Here's how the part is built. I have some questions about the finished solid (model axes, mm). Coordinates: 2 decimals unless noted, no trailing zeros. Order: outer loops, then holes, each group sorted by start corner. A loop starts at its lowest first (then second) coordinate and runs counter-clockwise, first axis right, second up. Notation, with made-up numbers: (5.5, -40) - (23.5, -40) arc R23 cw to (23.5, -31) - close; hole circle Ø1 at (-24, 38). An arc over 180 degrees is marked (long way). Answer as CSV lines item,"result". Start each with the question number.
Item 1: Imagine slicing it at A-A on x = 12.7. List the corners of the cut face in (y, z) for me, and give its area (3 significant figures).
Item 2: I need wall thicknesses on line 1 (Y direction, x = 12.7, z = 139); line 2 (X direction, y = 23.25, z = 264); line 3 (X direction, y = 16.75, z = 201) (3 decimals). Which ranges of each line are inside material? Lowest first, please.
Item 3: I'm going to push flat-ended pins straight in: pin 1 (5 mm diameter, centred on x = 12, z = 168.5, fed in from +Y); pin 2 (3 mm diameter, centred on y = 12.5, z = 186.5, fed in from +X); pin 3 (1.8 mm diameter, centred on y = 11.5, z = 166, fed in from -X). Where does each tip first touch, or does it pass through?
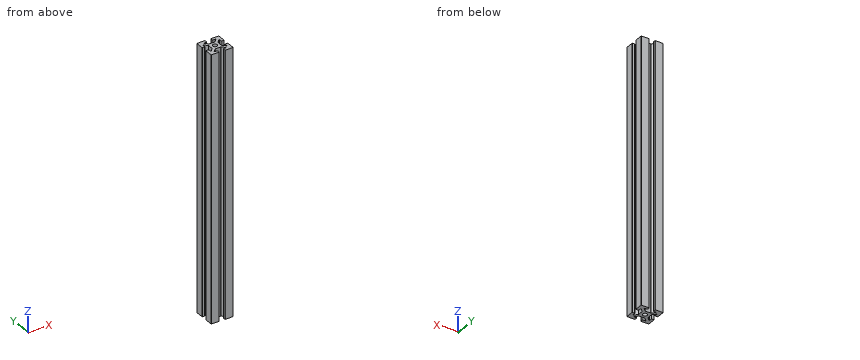
Autodesk Inventor part; units mm, degrees
ref_plane "YZ Plane" through (0, 0, 0) normal (1, 0, 0) x (0, 1, 0)
ref_plane "XZ Plane" through (0, 0, 0) normal (0, 1, 0) x (-1, 0, 0)
ref_plane "XY Plane" through (0, 0, 0) normal (0, 0, 1) x (1, 0, 0)
sketch "Sketch1" plane through (0, 0, 0) normal (0, 0, 1) x (1, 0, 0)
  line L0 (0, 0) -> (25.4, 0) construction
  line L1 (25.4, 0) -> (25.4, 25.4) construction
  line L2 (25.4, 25.4) -> (0, 25.4) construction
  line L3 (0, 25.4) -> (0, 0) construction
  line L4 (0, 25.4) -> (9.4615, 25.4) construction
  line L5 (9.4615, 25.4) -> (9.4615, 15.9385) construction
  line L6 (9.4615, 15.9385) -> (0, 15.9385) construction
  line L7 (0, 15.9385) -> (0, 25.4) construction
  line L8 (25.4, 25.4) -> (15.9385, 25.4) construction
  line L9 (15.9385, 25.4) -> (15.9385, 15.9385) construction
  line L10 (15.9385, 15.9385) -> (25.4, 15.9385) construction
  line L11 (25.4, 15.9385) -> (25.4, 25.4) construction
  line L12 (25.4, 0) -> (15.9385, 0) construction
  line L13 (15.9385, 0) -> (15.9385, 9.4615) construction
  line L14 (15.9385, 9.4615) -> (25.4, 9.4615) construction
  line L15 (25.4, 9.4615) -> (25.4, 0) construction
  line L16 (0, 0) -> (9.4615, 0) construction
  line L17 (9.4615, 0) -> (9.4615, 9.4615) construction
  line L18 (9.4615, 9.4615) -> (0, 9.4615) construction
  line L19 (0, 9.4615) -> (0, 0) construction
  circle A0 centre (12.7, 12.7) radius 2.5797
  line L20 (0, 25.4) -> (9.4615, 25.4)
  line L21 (9.4615, 25.4) -> (9.4615, 22.225)
  line L22 (0, 25.4) -> (0, 15.9385)
  line L23 (0, 15.9385) -> (3.175, 15.9385)
  line L24 (0, 0) -> (0, 9.4615)
  line L25 (0, 9.4615) -> (3.175, 9.4615)
  line L26 (0, 0) -> (9.4615, 0)
  line L27 (9.4615, 0) -> (9.4615, 3.175)
  line L28 (25.4, 0) -> (15.9385, 0)
  line L29 (25.4, 0) -> (25.4, 9.4615)
  line L30 (25.4, 9.4615) -> (22.225, 9.4615)
  line L31 (15.9385, 0) -> (15.9385, 3.175)
  line L32 (25.4, 25.4) -> (25.4, 15.9385)
  line L33 (25.4, 25.4) -> (15.9385, 25.4)
  line L34 (15.9385, 25.4) -> (15.9385, 22.225)
  line L35 (25.4, 15.9385) -> (22.225, 15.9385)
  line L36 (9.4615, 22.225) -> (5.2705, 22.225)
  line L37 (3.175, 15.9385) -> (3.175, 20.1295)
  line L38 (3.175, 9.4615) -> (3.175, 5.2705)
  line L39 (9.4615, 3.175) -> (5.2705, 3.175)
  line L40 (15.9385, 3.175) -> (20.1295, 3.175)
  line L41 (22.225, 9.4615) -> (22.225, 5.2705)
  line L42 (15.9385, 22.225) -> (20.1295, 22.225)
  line L43 (22.225, 15.9385) -> (22.225, 20.1295)
  line L44 (7.3422, 7.3422) -> (18.0578, 7.3422) construction
  line L45 (18.0578, 7.3422) -> (18.0578, 18.0578) construction
  line L46 (18.0578, 18.0578) -> (7.3422, 18.0578) construction
  line L47 (7.3422, 18.0578) -> (7.3422, 7.3422) construction
  line L48 (7.3422, 7.3422) -> (18.0578, 18.0578) construction
  line L49 (18.0578, 7.3422) -> (7.3422, 18.0578) construction
  line L50 (5.2705, 22.225) -> (9.4615, 18.0578)
  line L51 (3.175, 20.1295) -> (7.3422, 15.9385)
  line L52 (20.1295, 22.225) -> (15.9385, 18.0578)
  line L53 (22.225, 20.1295) -> (18.0578, 15.9385)
  line L54 (22.225, 5.2705) -> (18.0578, 9.4615)
  line L55 (20.1295, 3.175) -> (15.9385, 7.3422)
  line L56 (5.2705, 3.175) -> (9.4615, 7.3422)
  line L57 (3.175, 5.2705) -> (7.3422, 9.4615)
  line L58 (7.3422, 15.9385) -> (7.3422, 9.4615)
  line L59 (9.4615, 18.0578) -> (15.9385, 18.0578)
  line L60 (18.0578, 15.9385) -> (18.0578, 9.4615)
  line L61 (15.9385, 7.3422) -> (9.4615, 7.3422)
  dimension "d0" = 25.4
  dimension "d1" = 25.4
  dimension "d2" = 9.4615
  dimension "d3" = 9.4615
  dimension "d4" = 9.4615
  dimension "d5" = 9.4615
  dimension "d6" = 9.4615
  dimension "d7" = 9.4615
  dimension "d8" = 9.4615
  dimension "d9" = 9.4615
  dimension "d10" = 12.7
  dimension "d11" = 12.7
  dimension "d12" = 5.1594
  dimension "d13" = 3.175
  dimension "d14" = 3.175
  dimension "d15" = 3.175
  dimension "d16" = 3.175
  dimension "d17" = 3.175
  dimension "d18" = 3.175
  dimension "d19" = 3.175
  dimension "d20" = 3.175
  dimension "d21" = 4.191
  dimension "d22" = 4.191
  dimension "d23" = 4.191
  dimension "d24" = 4.191
  dimension "d25" = 4.191
  dimension "d26" = 4.191
  dimension "d27" = 4.191
  dimension "d28" = 4.191
  dimension "d29" = 10.7156
  dimension "d30" = 10.7156
extrude "Extrusion1" add sketch "Sketch1" along normal blind 304.8
fillet "Fillet1" radius 0.3969 35 edges at (9.4615, 25.4, 152.4) (9.4615, 22.225, 152.4) (5.2705, 22.225, 152.4) (9.4615, 18.0578, 152.4) (15.9385, 18.0578, 152.4) (20.1295, 22.225, 152.4) (15.9385, 22.225, 152.4) (15.9385, 25.4, 152.4) (25.4, 25.4, 152.4) (25.4, 15.9385, 152.4) (22.225, 15.9385, 152.4) (22.225, 20.1295, 152.4) (18.0578, 15.9385, 152.4) (18.0578, 9.4615, 152.4) (22.225, 5.2705, 152.4) (22.225, 9.4615, 152.4) (25.4, 9.4615, 152.4) (25.4, 0, 152.4) (15.9385, 0, 152.4) (15.9385, 3.175, 152.4) (20.1295, 3.175, 152.4) (15.9385, 7.3422, 152.4) (9.4615, 7.3422, 152.4) (5.2705, 3.175, 152.4) (9.4615, 3.175, 152.4) (9.4615, 0, 152.4) (0, 0, 152.4) (0, 9.4615, 152.4) (3.175, 5.2705, 152.4) (7.3422, 9.4615, 152.4) (7.3422, 15.9385, 152.4) (3.175, 20.1295, 152.4) (3.175, 15.9385, 152.4) (0, 15.9385, 152.4) (0, 25.4, 152.4)
properties part number "80-20 1x1"
Responses:
1,outline,"(7.34, 0) - (10.12, 0) - (10.12, 304.8) - (7.34, 304.8) - close; (15.28, 0) - (18.06, 0) - (18.06, 304.8) - (15.28, 304.8) - close"
1,area,"1,690 mm^2"
2,line 1,"y = 7.34 to 10.12, 15.28 to 18.06"
2,line 2,"x = 0 to 9.46, 15.94 to 25.4"
2,line 3,"x = 0 to 3.175, 6.535 to 18.865, 22.225 to 25.4"
3,pin 1,"stops at y = 18.08"
3,pin 2,"stops at x = 18.06"
3,pin 3,"stops at x = 7.34"
